Source: CAD feature listing. Evaluate the final solid. Frame: model axes, mm. Face numbers are marked on the shaded views. A direction names the side the tool comes from. Give positions to 0.01 mm unless a question says otherwise; leave off trailing zeros. Loops run counter-clockwise (first coordinate to the right, second up) from the corner with the lowest first, then second, coordinate; pieces in that order, holes last. Notation, with made-up numbers: M 72,-34.5 L 128,-34.5 A21 ccw 128,-21.5 Z; hole C 21,30.25 d10. An arc over 180 degrees is marked long. Answer in a Markdown table with one row per item.
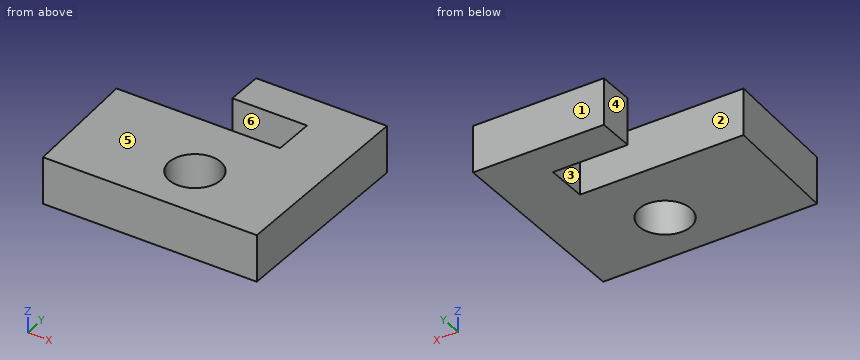
```python
from build123d import *

# Parameters (mm, degrees)
F1_DEPTH = 10
F3_D     = 11


with BuildPart() as f1:
    # F0 (on Top) → F1 (new body)
    with BuildSketch(Plane.XY):
        Polygon((-26.416933, 0), (-25.164945, -25.790939), (20.657791, -25.790939), (20.657791, 16.526233), (-7.386724, 16.526233), (-7.386724, 8.763911), (8.638713, 8.763911), (8.638713, 0), (0, 0), align=None)
    extrude(amount=F1_DEPTH)

    # F3 (through all)
    with Locations(Plane.XY.offset(10)):
        with Locations((0, -14.57391)):
            Hole(F3_D / 2)


solid = f1.part
```
1) Material intervals for L1, parallel to Y at x = 0, z = 4; L2, parallel to Y at x = -7, z = 4; L3, parallel to Y at x = 2.5, z = 4, sorted ascending.
Reply:
| item | result |
|---|---|
| L1 | y = -25.79 to -20.07, -9.07 to 0, 8.76 to 16.53 |
| L2 | y = -25.79 to 0, 8.76 to 16.53 |
| L3 | y = -25.79 to -19.47, -9.67 to 0, 8.76 to 16.53 |
2) Section B-B, the plane y = -16. Return loops of the section in (x, z), then the cut area to 3 significant figures.
Reply:
| item | result |
|---|---|
| outline | M -25.64,0 L -5.31,0 L -5.31,10 L -25.64,10 Z; M 5.31,0 L 20.66,0 L 20.66,10 L 5.31,10 Z |
| area | 357 mm² |
3) Set-up query: the marked faces 5 and 6. Return all of +Z, -Z, +X, -X, +Y, -Y with unobstructed straight access to the full face (end or side cutting, diameter ignored); none if empty.
Reply:
| item | result |
|---|---|
| face 5 | +Z, +X, -X, +Y, -Y |
| face 6 | +Z, -Z, -X |
4) Pull-direction query (Y, two-part tool) for the marked faces 1, 2, 3 and 4; classes: released by +Y, released by -Y, zero draft, split by the parting line, or undercut.
Reply:
| item | result |
|---|---|
| face 1 | released by +Y |
| face 2 | undercut |
| face 3 | undercut |
| face 4 | zero draft |
5) Section C-C, the plane z = 3.5. Return loops of the section in (x, y), then the cut area to 3 significant figures.
Reply:
| item | result |
|---|---|
| outline | M -26.42,0 L -25.16,-25.79 L 20.66,-25.79 L 20.66,16.53 L -7.39,16.53 L -7.39,8.76 L 8.64,8.76 L 8.64,0 Z; hole C 0,-14.57 d11 |
| area | 1,430 mm² |
6) Pin query (flat end, axial travel): pin 1 Ø2.5 at (y, z) = (13.5, 3) entering from -X; pin 2 Ø1.5 at (y, z) = (5, 4) entering from -X; pin 3 Ø6 at (x, y) = (-15, -20.5) entering from -Z; pin 4 Ø1.5 at (y, z) = (-11.5, 2) entering from -X. Return the tip coordinate at first contact, or that it passes through.
Reply:
| item | result |
|---|---|
| pin 1 | stops at x = -7.39 |
| pin 2 | stops at x = 8.64 |
| pin 3 | stops at z = 0 |
| pin 4 | stops at x = -25.9 |
7) Section A-A, the plane x = 0. Return loops of the section in (y, z), then the cut area to 3 significant figures.
Reply:
| item | result |
|---|---|
| outline | M -25.79,0 L -20.07,0 L -20.07,10 L -25.79,10 Z; M -9.07,0 L 0,0 L 0,10 L -9.07,10 Z; M 8.76,0 L 16.53,0 L 16.53,10 L 8.76,10 Z |
| area | 226 mm² |
8) Section D-D, the plane y = 14.5. Return loops of the section in (x, z).
Reply:
| item | result |
|---|---|
| outline | M -7.39,0 L 20.66,0 L 20.66,10 L -7.39,10 Z |
